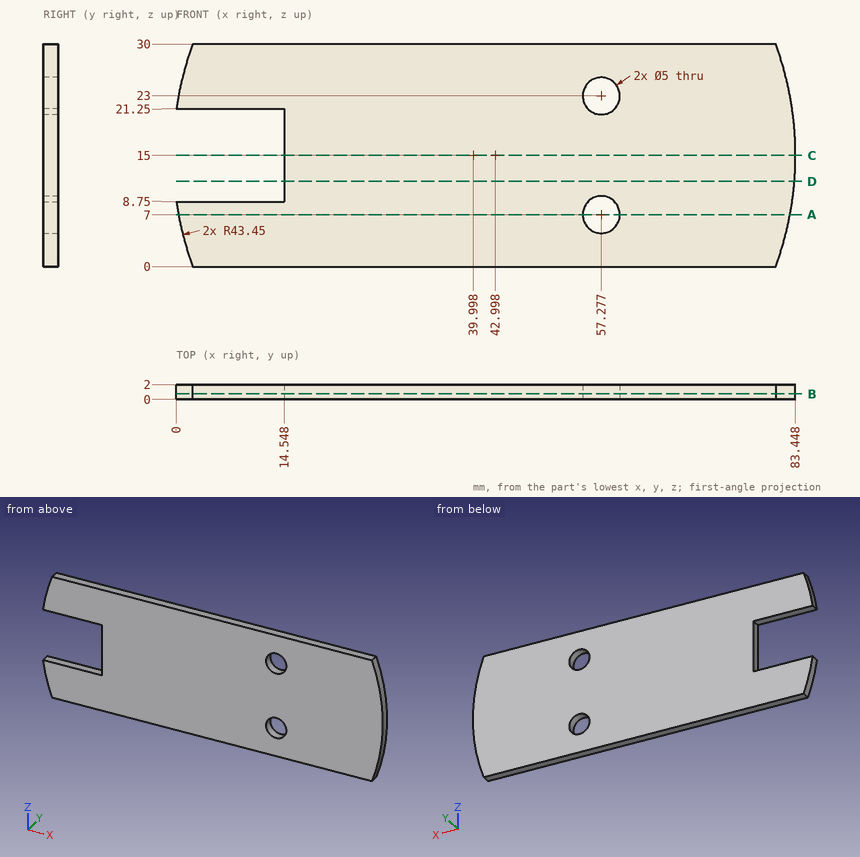
Input: dimensioned drawing with shaded views. Units: mm. Origin: part minimum x, y, z. Give positions to 0.01 mm unless a question says otherwise; leave off trailing zeros. Loops run counter-clockwise (first coordinate to the right, second up) from the corner with the lowest first, then second, coordinate; pieces in that order, holes last. Notation, with made-up numbers: (17.5, 64.25) -> (63.5, 64.25) arc R23 ccw to (63.5, 80.25) -> close; hole circle Ø2 at (19.25, 84). An arc over 180 degrees is marked (long way). Use a Markdown table: item, result. Add a question column.
1) Section query A-A, the plane z = 7. Return the cut outline in (x, y) (1 decimal), then the cut area to 3 significant figures.
2) Section query C-C, the plane z = 15. Return the cut outline in (x, y), then the cut area to 3 significant figures.
3) Line query: line 1 along Z through (x, y) = (59.5, 0.7) (1 decimal); line 2 along Z through (x, y) = (10.5, 0.9); line 3 along X through (y, z) = (0.4, 7) (1 decimal). Output: solid intervals per line, ascending. Write a range as [from, to].
4) First-contact query: pin 1 (1 mm diameter, centred on y = 1.5, z = 18, fed in from -X). Flat tip, straight axial feed; report the tip coordinate or a pass-through.
5) Section query D-D, the plane z = 11.5. Return the cut outline in (x, y).
6) Section query B-B, the plane y = 0.75. Return the cut outline in (x, z).
Numbers:
| question | item | result |
|---|---|---|
| 1 | outline | (0.3, 0) -> (54.8, 0) -> (54.8, 2) -> (0.3, 2) -> close; (59.8, 0) -> (82.7, 0) -> (82.7, 2) -> (59.8, 2) -> close |
| 1 | area | 155 mm2 |
| 2 | outline | (14.55, 0) -> (83.45, 0) -> (83.45, 2) -> (14.55, 2) -> close |
| 2 | area | 138 mm2 |
| 3 | line 1 | z = [0, 5.9], [8.1, 21.9], [24.1, 30] |
| 3 | line 2 | z = [0, 8.75], [21.25, 30] |
| 3 | line 3 | x = [0.3, 54.8], [59.8, 82.7] |
| 4 | pin 1 | stops at x = 14.55 |
| 5 | outline | (14.55, 0) -> (83.31, 0) -> (83.31, 2) -> (14.55, 2) -> close |
| 6 | outline | (0, 8.75) arc R43.45 ccw to (2.22, 0) -> (80.78, 0) arc R43.45 ccw to (80.78, 30) -> (2.22, 30) arc R43.45 ccw to (0, 21.25) -> (14.55, 21.25) -> (14.55, 8.75) -> close; hole circle Ø5 at (57.28, 7); hole circle Ø5 at (57.28, 23) |
